Input: part model. Units: mm. Frame: model coordinates. Face numbers are marked on the shaded views. A direction names the side the tool comes from. Give positions to 0.01 mm unless a question says otherwise; leave off trailing zeros. Write each loop counter-clockwise with the first axis right and the second up, starting at its lowest first coordinate (ties: lowest second). Pieces come first, ordered by that corner, then holes. Notation, with made-up numbers: (40, 24) -> (48, 24) arc R19 ccw to (48, 43) -> close; hole circle Ø2 at (-27, 75). An arc over 180 degrees is marked (long way). Return JSON: item names as keys, results as strings. Group by question number.
Item 1: Pin query (flat end, axial travel): P1, Ø2.5, axis at x = 1.5, y = 1.5, coming from the -Z side; P2, Ø3, axis at x = 8.5, y = 2.5, coming from the +Z side. Return the tip coordinate at first contact, or that it passes through.
Item 2: Set-up query: the marked faces 4 and 5. Return all of +Z, -Z, +X, -X, +Y, -Y with unobstructed straight access to the full face (end or side cutting, diameter ignored); none if empty.
Item 3: Section A-A, the plane z = 0.65. Return loops of the section in (x, y).
Item 4: Section B-B, the plane x = 0. Return loops of the section in (y, z).
Item 5: Mould query, pull axis Y, two halves, no side actions, for the marked faces 1, 2 and 3. Classes: released by +Y, released by -Y, zero draft, split by the parting line, or undercut.
Item 6: Line query: line 1 (X direction, y = 2.6, z = 0.45); line 2 (Y direction, x = 0, z = 4); line 3 (X direction, y = 0.45, z = 1.15). Output: solid intervals per line, ascending. Write a range as [from, to].
Item 7: Section C-C, the plane x = 2.75. Return loops of the section in (y, z), then the cut area to 3 significant figures.
Item 8: Section D-D, the plane z = 4.1. Return loops of the section in (x, y), then the cut area to 3 significant figures.
from build123d import *

# Parameters (mm, degrees)
SKETCH1_W           = 22
SKETCH1_H           = 5
SKETCH1_R           = 1.25
BOSS_EXTRUDE1_DEPTH = 5
SKETCH2_W           = 13
SKETCH2_H           = 3
CUT_EXTRUDE1_DEPTH  = 14.076696831
FILLET1_R           = 1
FILLET2_R           = 0.5
FILLET3_R           = 0.1


with BuildPart() as part:
    # Sketch1 → Boss-Extrude1 (new body)
    with BuildSketch(Plane.XY):
        with Locations((0, 2.5)):
            Rectangle(SKETCH1_W, SKETCH1_H)
        with Locations((8.5, 2.5)):
            Circle(SKETCH1_R, mode=Mode.SUBTRACT)
        with Locations((0, 2.5)):
            Circle(SKETCH1_R, mode=Mode.SUBTRACT)
        with Locations(Location((-8.5, 2.5, 0), (0, 0, 180))):
            Circle(SKETCH1_R, mode=Mode.SUBTRACT)
    extrude(amount=BOSS_EXTRUDE1_DEPTH)

    # Sketch2 → Cut-Extrude1 (cut, through all)
    with BuildSketch(Plane(origin=(0, 5, 0), x_dir=(1, 0, 0), z_dir=(0, 1, 0))):
        with Locations((0, -1.5)):
            Rectangle(SKETCH2_W, SKETCH2_H)
    extrude(amount=-CUT_EXTRUDE1_DEPTH, mode=Mode.SUBTRACT)

    # Fillet1
    fillet1_edges = [part.edges().sort_by_distance(p)[0] for p in [
        (-6.5, 2.5, 3),
        (6.5, 2.5, 3),
    ]]
    fillet(fillet1_edges, radius=FILLET1_R)

    # Fillet2
    fillet2_edges = [part.edges().sort_by_distance(p)[0] for p in [
        (11, 2.5, 5),
        (-11, 2.5, 5),
    ]]
    fillet(fillet2_edges, radius=FILLET2_R)

    # Fillet3
    fillet3_edges = [part.edges().sort_by_distance(p)[0] for p in [
        (-7.25, 2.5, 5),
        (7.25, 2.5, 5),
        (-1.25, 2.5, 5),
        (-8.75, 5, 0),
        (8.75, 0, 0),
        (-6.5, 0, 1),
        (-6.5, 5, 1),
        (6.5, 5, 1),
        (6.5, 0, 1),
        (0, 5, 3),
        (8.75, 5, 0),
        (0, 0, 3),
        (6.207106781, 5, 2.707106781),
        (6.207106781, 0, 2.707106781),
        (-6.207106781, 5, 2.707106781),
        (-6.207106781, 0, 2.707106781),
        (-8.75, 0, 0),
        (0, 0, 5),
        (0, 5, 5),
        (11, 0, 2.25),
        (-11, 0, 2.25),
        (10.853553391, 0, 4.853553391),
        (-10.853553391, 0, 4.853553391),
        (-11, 5, 2.25),
        (11, 5, 2.25),
        (10.853553391, 5, 4.853553391),
        (-10.853553391, 5, 4.853553391),
    ]]
    fillet(fillet3_edges, radius=FILLET3_R)


solid = part.part
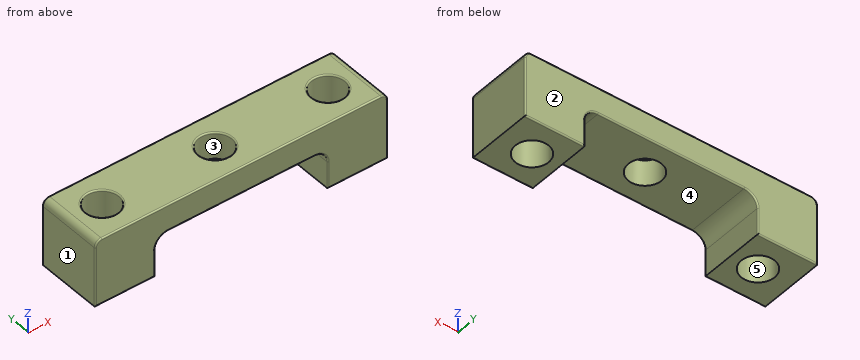
Answer below:
{
 "1": {"P1": "stops at z = 3", "P2": "stops at z = 5"},
 "2": {"face 4": "-Z, +Y, -Y", "face 5": "+Z, -Z"},
 "3": {"outline": "(-11, 0.1) arc R0.1 ccw to (-10.9, 0) -> (-6.6, 0) arc R0.1 ccw to (-6.5, 0.1) -> (-6.5, 4.9) arc R0.1 ccw to (-6.6, 5) -> (-10.9, 5) arc R0.1 ccw to (-11, 4.9) -> close; (6.5, 0.1) arc R0.1 ccw to (6.6, 0) -> (10.9, 0) arc R0.1 ccw to (11, 0.1) -> (11, 4.9) arc R0.1 ccw to (10.9, 5) -> (6.6, 5) arc R0.1 ccw to (6.5, 4.9) -> close; hole circle Ø2.5 at (-8.5, 2.5); hole circle Ø2.5 at (8.5, 2.5)"},
 "4": {"outline": "(0, 3.1) arc R0.1 ccw to (0.1, 3) -> (1.25, 3) -> (1.25, 4.9) arc R0.1 ccw to (1.15, 5) -> (0.1, 5) arc R0.1 ccw to (0, 4.9) -> close; (3.75, 3) -> (4.9, 3) arc R0.1 ccw to (5, 3.1) -> (5, 4.9) arc R0.1 ccw to (4.9, 5) -> (3.85, 5) arc R0.1 ccw to (3.75, 4.9) -> close"},
 "5": {"face 1": "zero draft", "face 2": "released by +Y", "face 3": "undercut"},
 "6": {"line 1": "x = [-11, -9.75], [-7.25, -6.5], [6.5, 7.25], [9.75, 11]", "line 2": "y = [0, 1.25], [3.75, 5]", "line 3": "x = [-11, -6.5], [6.5, 11]"},
 "7": {"outline": "(0, 3.1) arc R0.1 ccw to (0.1, 3) -> (4.9, 3) arc R0.1 ccw to (5, 3.1) -> (5, 4.9) arc R0.1 ccw to (4.9, 5) -> (0.1, 5) arc R0.1 ccw to (0, 4.9) -> close", "area": "9.99 mm2"},
 "8": {"outline": "(-11, 0.1) arc R0.1 ccw to (-10.9, 0) -> (10.9, 0) arc R0.1 ccw to (11, 0.1) -> (11, 4.9) arc R0.1 ccw to (10.9, 5) -> (-10.9, 5) arc R0.1 ccw to (-11, 4.9) -> close; hole circle Ø2.5 at (-8.5, 2.5); hole circle Ø2.5 at (0, 2.5); hole circle Ø2.5 at (8.5, 2.5)", "area": "95.3 mm2"}
}
